Design review of the part built by this model. Coordinates are the model's own, in mm. A direction names the side the tool comes from. Round coordinates to 2 decimals unless told otherwise and drop trailing zeros. Loops run counter-clockwise (first coordinate to the right, second up) from the corner with the lowest first, then second, coordinate; pieces in that order, holes last. Notation, with made-up numbers: (7, -25) -> (38, -25) arc R27 ccw to (38, 5) -> close; hole circle Ø7 at (36, 21.25). An arc over 180 degrees is marked (long way). Answer as CSV lines item,"result". Start each with the question number.
Autodesk Fusion 360 part; units mm, degrees
sketch "Esboço1" plane through (0, 0, 0) normal (0, 0, 1) x (1, 0, 0)
  circle A0 centre (0, 0) radius 9.5
  circle A1 centre (0, 0) radius 12.5
  line L0 (-30, 22.0941) -> (-30, -26.9412) construction
  line L1 (-41.3447, -13.125) -> (30, -13.125) construction
  line L2 (-30, -13.125) -> (-9.0024, 8.6722)
  line L3 (-30, -13.125) -> (-30, -15)
  line L4 (-30, -15) -> (0, -15)
  line L5 (0, 0) -> (0, -30) construction
  line L6 (30, -13.125) -> (9.0024, 8.6722)
  line L7 (30, -13.125) -> (30, -15)
  line L8 (30, -15) -> (0, -15)
  dimension "d1" = 25
  dimension "d2" = 19
  dimension "d3" = 30
  dimension "d4" = 13.125
  dimension "d6" = 1.875
extrude "Extrusão1" add sketch "Esboço1" along normal blind 6.5
sketch "Esboço2" plane through (0, -15, 0) normal (0, -1, 0) x (1, 0, 0)
  line L0 (-30, 0) -> (30, 0)
  line L1 (30, 0) -> (30, 6.5)
  line L2 (30, 6.5) -> (-30, 6.5)
  line L3 (-30, 6.5) -> (-30, 0)
  line L4 (0, 0) -> (0, 15) construction
  line L5 (-20, 3.25) -> (20, 3.25) construction
  circle A0 centre (-20, 3.25) radius 1.5
  circle A1 centre (20, 3.25) radius 1.5
  dimension "d9" = 20
  dimension "d10" = 20
  dimension "d11" = 3.25
  dimension "d12" = 3
extrude "Extrusão2" cut sketch "Esboço2" against normal blind 8 contours A0 | A1
thread "Rosca1"
Q1. Add section C-C, the plane y = -10.75. Give the boundary of the cut face in (x, z).
Q2. Add section A-A, the plane y = -6. Give the boundary of the cut face in (x, z).
Q3. Machinability: for faces 1 (the flat face through (0, -15, 3)), 2 (the flat face through (-20, -7, 3)), which of the approach directions +Z, -Z, +X, -X, +Y, -Y give a long, thin tool a straight path to every point of the face, cutting with its end or side? Answer none if there is none.
Q4. To check wall thickness, follow probe 1 along X at (y, z) = (-8.25, 4.25); probe 2 along X at (y, z) = (-9.75, 2); probe 3 along X at (y, z) = (3.5, 2.5). State the ranges of each line that lie inside material, in increasing order. Write a range as from..to.
Q5. Mouldability with a two-part tool opening along Z and no side actions: class faces 3 (the cylindrical face through (-21.5, -11.1, 3.3)), 4 (the flat face through (30, -14, 3)), 5 (the flat face through (0, -10, 6.5)) as pulls with the +Z half, pulls with the -Z half, needs draft (parallel to the pull), parting line crosses it, or undercut.
Q6. Add section D-D, the plane y = 2.25. Give the boundary of the cut face in (x, z), and give its area (3 significant figures).
Q7. Add section B-B, the plane x = 20. Give the boundary of the cut face in (y, z).
Q8. For pin 1 Ø1 at (y, z) = (-6.5, 3) entering from +X; pin 2 Ø2.5 at (x, z) = (-20, 3.25) entering from +Y; pin 3 Ø1.5 at (x, z) = (20, 3) entering from -Y, all flat-tipped, find the tip position at first contact; note any pin that passes through.
Worked answers:
1,outline,"(-27.71, 0) -> (27.71, 0) -> (27.71, 6.5) -> (-27.71, 6.5) -> close; hole circle Ø3 at (-20, 3.25); hole circle Ø3 at (20, 3.25)"
2,outline,"(-23.14, 0) -> (-7.37, 0) -> (-7.37, 6.5) -> (-23.14, 6.5) -> close; (7.37, 0) -> (23.14, 0) -> (23.14, 6.5) -> (7.37, 6.5) -> close"
3,face 1,"+Z, -Z, +X, -X, -Y"
3,face 2,"-Y"
4,probe 1,"x = -25.3..-21.12, -18.88..-4.71, 4.71..18.88, 21.12..25.3"
4,probe 2,"x = -26.75..-20.83, -19.17..19.17, 20.83..26.75"
4,probe 3,"x = -13.98..-8.83, 8.83..13.98"
5,face 3,"undercut"
5,face 4,"needs draft"
5,face 5,"pulls with the +Z half"
6,outline,"(-15.19, 0) -> (-9.23, 0) -> (-9.23, 6.5) -> (-15.19, 6.5) -> close; (9.23, 0) -> (15.19, 0) -> (15.19, 6.5) -> (9.23, 6.5) -> close"
6,area,"77.5 mm^2"
7,outline,"(-15, 0) -> (-2.74, 0) -> (-2.74, 6.5) -> (-15, 6.5) -> (-15, 4.75) -> (-7, 4.75) -> (-7, 1.75) -> (-15, 1.75) -> close"
8,pin 1,"stops at x = 24.1"
8,pin 2,"stops at y = -1.45"
8,pin 3,"stops at y = -7"
